CAD build for the part. Positions are in the model's coordinates, mm. A direction names the side the tool comes from. Coordinates: 2 decimals unless noted, no trailing zeros. Order: outer loops, then holes, each group sorted by start corner. A loop starts at its lowest first (then second) coordinate and runs counter-clockwise, first axis right, second up. Notation, with made-up numbers: (57, 74.25) - (83, 74.25) arc R6 cw to (83, 83.25) - close; hole circle Ø7 at (64.25, -31). An arc over 180 degrees is marked (long way). Use one line per item in the form item = value.
```python
from build123d import *

# Parameters (mm, degrees)
SKETCH_1_W          = 50
SKETCH_1_H          = 13
EXTRUDE_1_DEPTH     = 8
SKETCH_2_R          = 6.35
EXTRUDE_2_DEPTH     = 55
SKETCH_3_W          = 50
SKETCH_3_H          = 3.2
CUT_EXTRUDE_1_DEPTH = 5


with BuildPart() as part:
    # 草图1 → 凸台-拉伸1 (new body)
    with BuildSketch(Plane(origin=(0, 0, 0), x_dir=(1, 0, 0), z_dir=(0, 1, 0))):
        Rectangle(SKETCH_1_W, SKETCH_1_H)
    extrude(amount=EXTRUDE_1_DEPTH)

    # 草图2 → 凸台-拉伸2 (add)
    with BuildSketch(Plane.XZ):
        with Locations(Location((0, 0, 0), (0, 0, 270))):
            Circle(SKETCH_2_R)
    extrude(amount=EXTRUDE_2_DEPTH)

    # 草图3 → 切除-拉伸1 (cut)
    with BuildSketch(Plane(origin=(0, 8, 0), x_dir=(1, 0, 0), z_dir=(0, 1, 0))):
        Rectangle(SKETCH_3_W, SKETCH_3_H)
    extrude(amount=-CUT_EXTRUDE_1_DEPTH, mode=Mode.SUBTRACT)


solid = part.part
```
Item 1: Cut at C-C, the plane y = -50. Write the cut outline in (x, z), plus the area to 3 significant figures.
Derived:
outline = circle Ø12.7 at (0, 0)
area = 127 mm²
Item 2: Cut at B-B, the plane x = 0. Write the cut outline in (y, z).
Derived:
outline = (-55, -6.35) - (0, -6.35) - (0, -6.5) - (8, -6.5) - (8, -1.6) - (3, -1.6) - (3, 1.6) - (8, 1.6) - (8, 6.5) - (0, 6.5) - (0, 6.35) - (-55, 6.35) - close
Item 3: Drop flat-ended pins along their axis: pin 1 (2.5 mm diameter, centred on x = -8.5, z = 0, fed in from +Y); pin 2 (5 mm diameter, centred on x = 9, z = 0.5, fed in from -Y); pin 3 (1.5 mm diameter, centred on y = -31.5, z = 3, fed in from +X). Give the stop position or say it passes through.
Derived:
pin_1 = 3
pin_2 = 0
pin_3 = 5.94
Item 4: Two-plate mould, pull along Z, no slides. Class faces 1 (the face through (0, 8, 4)), 2 (the face through (0, 6, 1.6)), 3 (the face through (-3.86, -27.12, 5.04)), 4 (the face through (0, 3, 0)): +Z half, -Z half, draft (parallel to the pull), parting line (faces both ways), or undercut.
Derived:
face_1 = draft
face_2 = undercut
face_3 = parting line
face_4 = undercut
Item 5: Cut at D-D, the plane z = 4.5. Write the cut outline in (x, y).
Derived:
outline = (-25, 0) - (-4.48, 0) - (-4.48, -55) - (4.48, -55) - (4.48, 0) - (25, 0) - (25, 8) - (-25, 8) - close
Item 6: Drill centre lines: line 1 (Y direction, x = -13, z = -4.25); line 2 (Y direction, x = 15.5, z = -1.25); line 3 (X direction, y = -14.5, z = 5.5). Where is each one in solid material? Low to high. Write a range as [from, to].
Derived:
line_1 = [0, 8]
line_2 = [0, 3]
line_3 = [-3.17, 3.17]
Item 7: 3-axis set-ups, long thin cutter, end or side, ignore diameter. For faces 5 (the face through (25, 2, 0)), 6 (the face through (0, 6, -1.6)): which of +Z, -Z, +X, -X, +Y, -Y reach the whole face in a straight line?
Derived:
face_5 = +Z, -Z, +X, +Y, -Y
face_6 = +X, -X, +Y
Item 8: Cut at A-A, the plane z = 0. Write the cut outline in (x, y).
Derived:
outline = (-25, 0) - (-6.35, 0) - (-6.35, -55) - (6.35, -55) - (6.35, 0) - (25, 0) - (25, 3) - (-25, 3) - close
